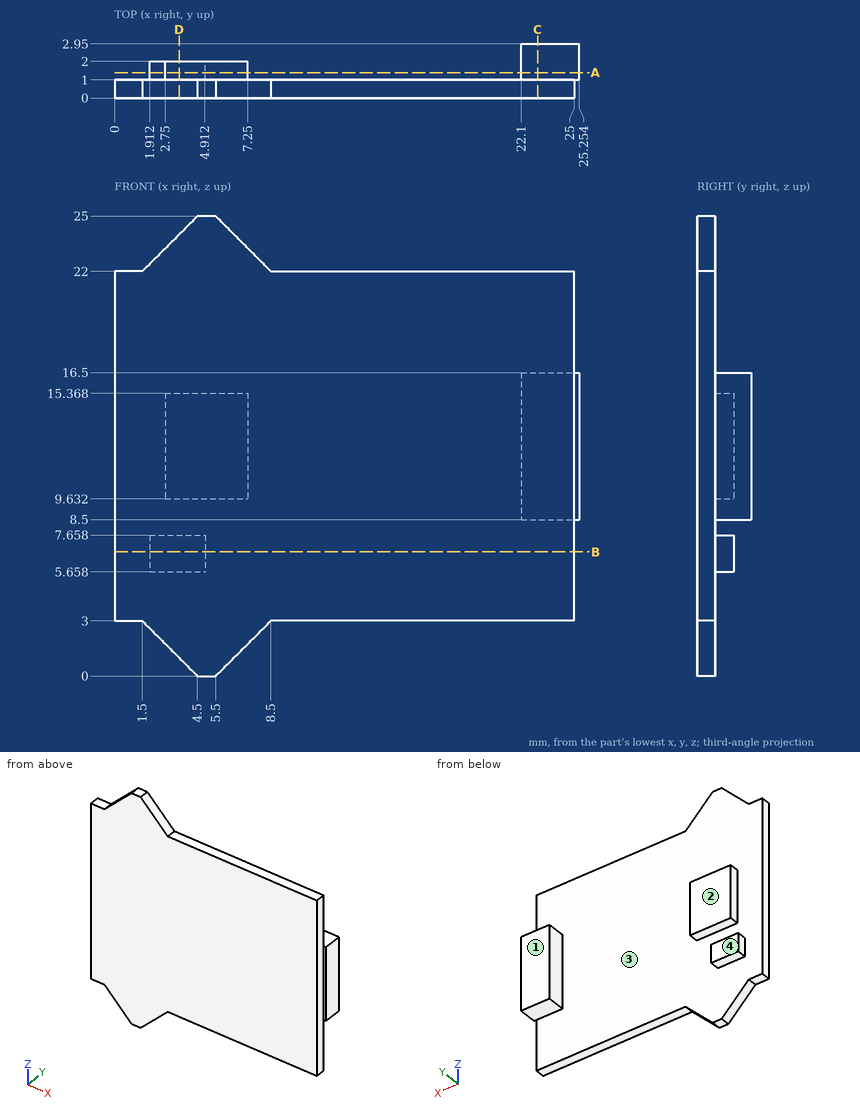
Source: three-view drawing plus pictorial views. Frame: mm from the lowest corner of the part. A direction names the side the tool comes from. Give positions to 0.01 mm unless a question says otherwise; leave off trailing zeros. Write each loop counter-clockwise with the first axis right and the second up, starting at its lowest first coordinate (ties: lowest second). Pieces come first, ordered by that corner, then holes. Notation, with made-up numbers: (-2, -4.75) - (31, -4.75) arc R17 cw to (31, 8.25) - close; hole circle Ø4 at (4, 15). An arc over 180 degrees is marked (long way). Write item = value, one per line. Start each with the question number.
Q1. Cut plane C-C, the plane x = 23. Return loops of the section in (y, z).
Q2. Draft query along X for the marked faces 3 and 4. Return one class per face: +X half, -X half, draft (parallel to the pull), parting line (faces both ways), or undercut.
Q3. Pin query (flat end, axial travel): pin 1 Ø0.5 at (y, z) = (1.5, 13.5) entering from -X; pin 2 Ø0.6 at (x, y) = (23.5, 2) entering from -Z; pin 3 Ø1.1 at (x, y) = (20.5, 0.5) entering from -Z. Return the tip coordinate at first contact, or that it passes through.
Q4. Reachability of the marked faces 1 and 2 from +Z, -Z, +X, -X, +Y, -Y: full face, straight path, thin tool, end or side. Return the list, or none.
Q5. Cut plane A-A, the plane y = 1.4. Give the number of separate pieces and of enclosed holes in the cut face.
Q6. Cut plane D-D, the plane x = 3.5. Return loops of the section in (y, z).
Q7. Material intervals for probe 1 along Y at (x, z) = (9, 16); probe 2 along Z at (x, y) = (18.5, 0.2); probe 3 along Z at (x, y) = (6.5, 1.9), sorted ascending.
Q8. Cut plane B-B, the plane z = 6.75. Return loops of the section in (x, y).
Computed values:
q1.outline = (0, 3) - (1, 3) - (1, 8.5) - (2.95, 8.5) - (2.95, 16.5) - (1, 16.5) - (1, 22) - (0, 22) - close
q2.face_3 = undercut
q2.face_4 = draft
q3.pin_1 = 2.75
q3.pin_2 = 8.5
q3.pin_3 = 3
q4.face_1 = +Z, -Z, +X, -X, +Y
q4.face_2 = +Z, -Z, -X, +Y
q5.separate_pieces = 3
q5.enclosed_holes = 0
q6.outline = (0, 1) - (1, 1) - (1, 5.66) - (2, 5.66) - (2, 7.66) - (1, 7.66) - (1, 9.63) - (2, 9.63) - (2, 15.37) - (1, 15.37) - (1, 24) - (0, 24) - close
q7.probe_1 = 0 to 1
q7.probe_2 = 3 to 22
q7.probe_3 = 9.63 to 15.37
q8.outline = (0, 0) - (25, 0) - (25, 1) - (4.91, 1) - (4.91, 2) - (1.91, 2) - (1.91, 1) - (0, 1) - close
